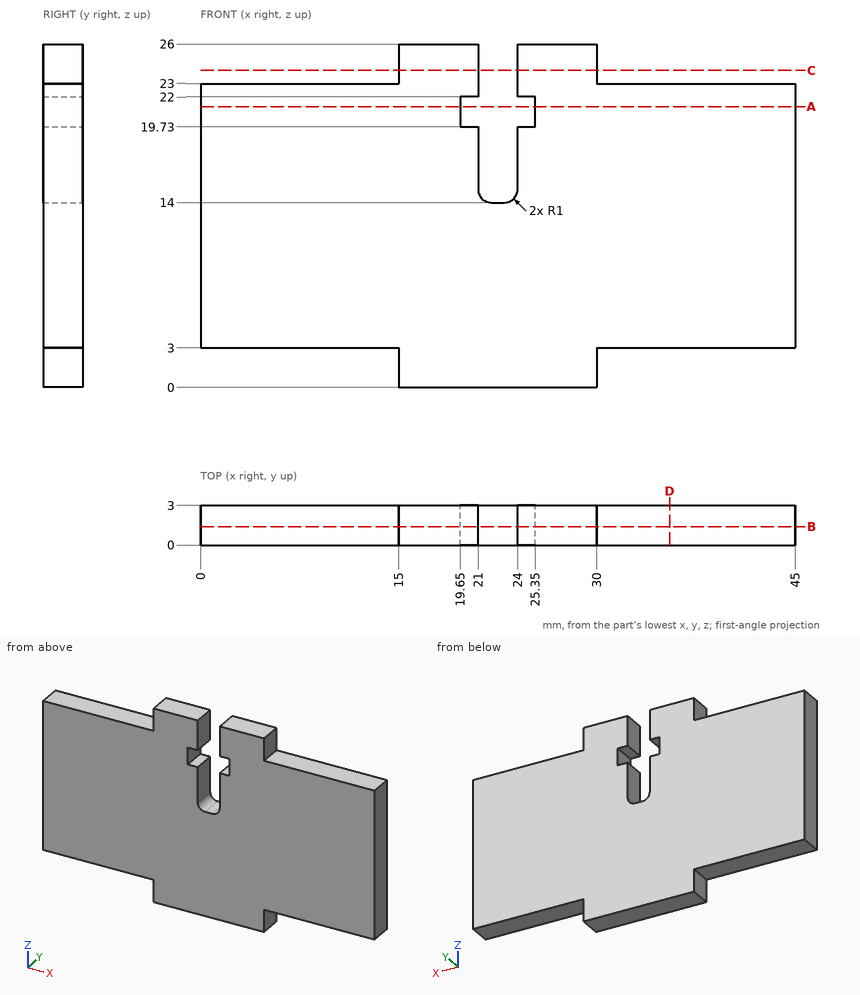
Design review of the part shown in the three views and the two pictorial views. Dimensions are in mm from the part's minimum x, y and z. Round coordinates to 2 decimals unless told otherwise and drop trailing zeros. Order: outer loops, then holes, each group sorted by start corner. A loop starts at its lowest first (then second) coordinate and runs counter-clockwise, first axis right, second up. Notation, with made-up numbers: M 9.25,22 L 66.25,22 A29 ccw 66.25,48 Z; hole C -23.75,87 d2. An arc over 180 degrees is marked long. Put each result on its own line as item: value.
Q1. Insertion check: pin 1 Ø1.5 at (x, y) = (10, 1) entering from +Z; pin 2 Ø0.9 at (y, z) = (1.5, 25) entering from -X; pin 3 Ø0.9 at (x, y) = (40, 2) entering from -Z. Each pin has a flat end and moves straight along its axis. Give the tip position at first contact, or say it passes through.
Reported:
pin 1: z = 23
pin 2: x = 15
pin 3: z = 3
Q2. Consider section C-C (z = 24). State the section outline as (x, y) points.
Reported:
outline: M 15,0 L 21,0 L 21,3 L 15,3 Z; M 24,0 L 30,0 L 30,3 L 24,3 Z
Q3. Consider section A-A (z = 21.25). State the section outline as (x, y) points, and give its area (3 significant figures).
Reported:
outline: M 0,0 L 19.65,0 L 19.65,3 L 0,3 Z; M 25.35,0 L 45,0 L 45,3 L 25.35,3 Z
area: 118 mm²
Q4. Consider section B-B (y = 1.4). State the section outline as (x, z) points.
Reported:
outline: M 0,3 L 15,3 L 15,0 L 30,0 L 30,3 L 45,3 L 45,23 L 30,23 L 30,26 L 24,26 L 24,22 L 25.35,22 L 25.35,19.73 L 24,19.73 L 24,15 A1 cw 23,14 L 22,14 A1 cw 21,15 L 21,19.73 L 19.65,19.73 L 19.65,22 L 21,22 L 21,26 L 15,26 L 15,23 L 0,23 Z
Q5. Consider section D-D (x = 35.5). State the section outline as (y, z) points, and give its area (3 significant figures).
Reported:
outline: M 0,3 L 3,3 L 3,23 L 0,23 Z
area: 60.0 mm²
Q6. To check wall thickness, follow line 1 (Z direction, x = 20.5, y = 0.4); line 2 (X direction, y = 1.15, z = 22.25); line 3 (X direction, y = 0.1, z = 24). State the ranges of each line that lie inside material, in increasing order.
Reported:
line 1: 0 to 19.73, 22 to 26
line 2: 0 to 21, 24 to 45
line 3: 15 to 21, 24 to 30
